Model file for the job. Use its own axes, mm. Face numbers are marked on the shaded views. A direction names the side the tool comes from. Coordinates: 2 decimals unless noted, no trailing zeros. Write each loop counter-clockwise with the first axis right and the second up, starting at its lowest first coordinate (ties: lowest second). Pieces come first, ordered by that corner, then holes. Notation, with made-up numbers: M 4,39 L 23,39 A29 ccw 23,76 Z; hole C 86,33.25 d11. An arc over 180 degrees is marked long. One line per question, with ' | ' between items. Start each with the question number.
(1) Flat gauge pins, fed straight in: pin 1 Ø1.5 at (y, z) = (3, 80.5) entering from -X; pin 2 Ø2 at (y, z) = (3, 45) entering from +X; pin 3 Ø1.2 at (y, z) = (1.5, 22.5) entering from +X. Where does each tip first touch, or does it go through?
(2) Wall check: probe 1 along Y at (x, z) = (4.5, 45.5); probe 2 along Z at (x, y) = (1.5, 3.5); probe 3 along Y at (x, z) = (5, 51). Give the ranges that are in metal, low to high.
(3) Cut at A-A (z = 45). Write the cut outline in (x, y).
(4) Cut at B-B (z = 69). Write the cut outline in (x, y).
(5) Tool access for the marked faces 1, 2, 3 and 4: list every direction of +Z, -Z, +X, -X, +Y, -Y with a clear straight run to the whole face (end or side of a thin tool).
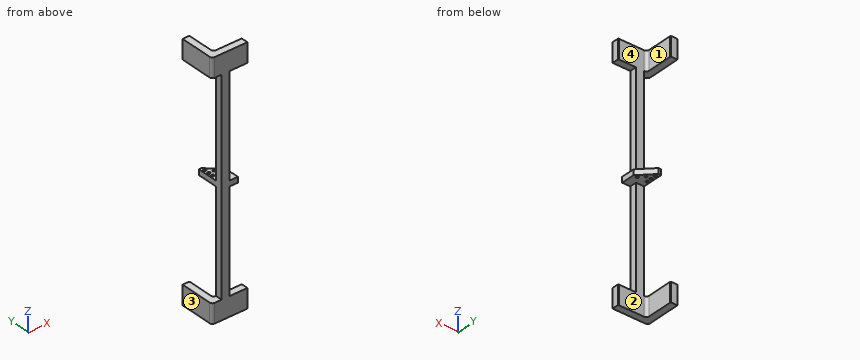
from build123d import *

# Parameters (mm, degrees)
PAD_DEPTH       = 7
FILLET_R        = 1
FILLET001_R     = 1
CHAMFER_SIZE    = 0.2
CHAMFER001_SIZE = 0.2
SKETCH001_W     = 3
SKETCH001_H     = 2.5
PAD001_DEPTH    = 76
PAD002_DEPTH    = 7
FILLET002_R     = 1
FILLET003_R     = 1
CHAMFER002_SIZE = 0.2
CHAMFER003_SIZE = 0.2
SKETCH003_W     = 10
SKETCH003_H     = 2
PAD003_DEPTH    = 3
CHAMFER004_SIZE = 5
SKETCH004_R     = 0.5
POCKET_DEPTH    = 46.001


with BuildPart() as part:
    # Sketch → Pad (new body)
    with BuildSketch(Plane.XY):
        Polygon((0, 0), (0, 13), (2.5, 13), (2.5, 2.5), (13, 2.5), (13, 0), align=None)
    extrude(amount=PAD_DEPTH)

    # Fillet
    fillet_edges = [part.edges().sort_by_distance(p)[0] for p in [
        (2.5, 2.5, 3.5),
    ]]
    fillet(fillet_edges, radius=FILLET_R)

    # Fillet001
    fillet001_edges = [part.edges().sort_by_distance(p)[0] for p in [
        (0, 0, 3.5),
    ]]
    fillet(fillet001_edges, radius=FILLET001_R)

    # Chamfer
    chamfer_edges = [part.edges().sort_by_distance(p)[0] for p in [
        (2.5, 13, 3.5),
    ]]
    chamfer(chamfer_edges, length=CHAMFER_SIZE)

    # Chamfer001
    chamfer001_edges = [part.edges().sort_by_distance(p)[0] for p in [
        (13, 2.5, 3.5),
    ]]
    chamfer(chamfer001_edges, length=CHAMFER001_SIZE)

    # Sketch001 → Pad001 (new body)
    with BuildSketch(Plane.XY.offset(7)):
        with Locations((5, 1.25)):
            Rectangle(SKETCH001_W, SKETCH001_H)
    extrude(amount=PAD001_DEPTH)

    # Sketch002 → Pad002 (new body)
    with BuildSketch(Plane.XY.offset(83)):
        Polygon((2.5, 2.5), (13, 2.5), (13, 0), (0, 0), (0, 13), (2.5, 13), align=None)
    extrude(amount=PAD002_DEPTH)

    # Fillet002
    fillet002_edges = [part.edges().sort_by_distance(p)[0] for p in [
        (0, 0, 86.5),
    ]]
    fillet(fillet002_edges, radius=FILLET002_R)

    # Fillet003
    fillet003_edges = [part.edges().sort_by_distance(p)[0] for p in [
        (2.5, 2.5, 86.5),
    ]]
    fillet(fillet003_edges, radius=FILLET003_R)

    # Chamfer002
    chamfer002_edges = [part.edges().sort_by_distance(p)[0] for p in [
        (2.5, 13, 86.5),
    ]]
    chamfer(chamfer002_edges, length=CHAMFER002_SIZE)

    # Chamfer003
    chamfer003_edges = [part.edges().sort_by_distance(p)[0] for p in [
        (13, 2.5, 86.5),
    ]]
    chamfer(chamfer003_edges, length=CHAMFER003_SIZE)

    # Sketch003 → Pad003 (new body, symmetric)
    with BuildSketch(Plane.YZ.offset(6.5)):
        with Locations((5, 45)):
            Rectangle(SKETCH003_W, SKETCH003_H)
    extrude(amount=PAD003_DEPTH, both=True)

    # Chamfer004
    chamfer004_edges = [part.edges().sort_by_distance(p)[0] for p in [
        (9.5, 10, 45),
    ]]
    chamfer(chamfer004_edges, length=CHAMFER004_SIZE)

    # Sketch004 → Pocket (cut, through all)
    with BuildSketch(Plane.XY.offset(46)):
        with Locations((4.5, 8.6)):
            Circle(SKETCH004_R)
        with Locations((4.5, 6.75)):
            Circle(SKETCH004_R)
        with Locations((4.5, 5)):
            Circle(SKETCH004_R)
        with Locations((6.35, 6.75)):
            Circle(SKETCH004_R)
        with Locations((8.1, 5)):
            Circle(SKETCH004_R)
    extrude(amount=-POCKET_DEPTH, mode=Mode.SUBTRACT)


solid = part.part
Filled in:
1) pin 1: x = 3.5 | pin 2: x = 9.5 | pin 3: x = 6.5
2) probe 1: 0 to 4.5, 5.5 to 6.25, 7.25 to 8.1, 9.1 to 10 | probe 2: 0 to 7, 83 to 90 | probe 3: 0 to 2.5
3) outline: M 3.5,0 L 9.5,0 L 9.5,5 L 4.5,10 L 3.5,10 Z; hole C 4.5,5 d1; hole C 4.5,6.75 d1; hole C 4.5,8.6 d1; hole C 6.35,6.75 d1; hole C 8.1,5 d1
4) outline: M 3.5,0 L 6.5,0 L 6.5,2.5 L 3.5,2.5 Z
5) face 1: +Z, -Z, +X, +Y | face 2: -Z, +X, +Y | face 3: +Z, -Z, -X, +Y, -Y | face 4: +Z, +X, +Y
